```python
from build123d import *

# Parameters (mm, degrees)
BOSS_EXTRUDE3_DEPTH = 159.5
SHELL1_T            = -2.5
SKETCH1_W           = 154.5
SKETCH1_H           = 67.5
CUT_EXTRUDE2_DEPTH  = 4
CUT_EXTRUDE1_REACH  = 161.5
SKETCH2_W           = 4
SKETCH2_H           = 26
SKETCH8_W           = 179.5
SKETCH8_H           = 111.610999554
SKETCH8_W_2         = 159.5
SKETCH8_H_2         = 91.610999554
CUT_EXTRUDE3_DEPTH  = 56.944109771
SKETCH10_W          = 31.5
SKETCH10_H          = 55
CUT_EXTRUDE4_DEPTH  = 2.5
BOSS_EXTRUDE4_DEPTH = 13
CUT_EXTRUDE5_DEPTH  = 3.302
SKETCH13_R          = 2.6
CUT_EXTRUDE6_DEPTH  = 2.5
BOSS_EXTRUDE5_DEPTH = 1.6
SKETCH15_R          = 4
SKETCH15_R_2        = 1.4
BOSS_EXTRUDE6_DEPTH = 3
CUT_EXTRUDE7_REACH  = 6.236
SKETCH15_2_R        = 1.4


with BuildPart() as part:
    # Sketch3 → Boss-Extrude3 (new body)
    with BuildSketch(Plane.YZ.offset(-81.169946448)):
        Polygon((37, 0), (50.833221776, -14.444444444), (7.499888442, -55.944109771), (-40.777777778, -5.53328871), (-35, 0), align=None)
    extrude(amount=BOSS_EXTRUDE3_DEPTH)

    # Shell1
    shell1_openings = [part.faces().sort_by_distance(p)[0] for p in [
        (-1.419946448, 1, 0),
    ]]
    offset(amount=SHELL1_T, openings=shell1_openings, kind=Kind.INTERSECTION)

    # Sketch1 → Cut-Extrude2 (cut)
    with BuildSketch(Plane.XY):
        with Locations((-1.419946448, 0.902066229)):
            Rectangle(SKETCH1_W, SKETCH1_H)
    extrude(amount=-CUT_EXTRUDE2_DEPTH, mode=Mode.SUBTRACT)

    # Sketch2 → Cut-Extrude1 (cut, up to next)
    with BuildSketch(Plane.ZY.offset(81.169946448), mode=Mode.PRIVATE) as cut_extrude1_sk1:
        with Locations((-15.25, -1.097933771)):
            Rectangle(SKETCH2_W, SKETCH2_H)
    cut_extrude1_tool1 = extrude(cut_extrude1_sk1.sketch, amount=-CUT_EXTRUDE1_REACH, mode=Mode.PRIVATE) & part.part
    add(cut_extrude1_tool1.solids().sort_by_distance((-81.169946, -1.097934, -15.25))[0], mode=Mode.SUBTRACT)

    # Sweep1: sweep along a path in Sketch6
    with BuildLine(Plane.XY.offset(-1.8)) as sweep1_path:
        Line((-78.669946448, 34.652066229), (75.830053552, 34.652066229))
        Line((75.830053552, 34.652066229), (75.830053552, -32.847933771))
        Line((75.830053552, -32.847933771), (-78.669946448, -32.847933771))
        Line((-78.669946448, -32.847933771), (-78.669946448, 34.652066229))
    # Sketch7 → Sweep1 (sweep)
    with BuildSketch(Plane.ZY.offset(-75.830053552)):
        Polygon((-1.356838972, 35.114808383), (-2.636411987, 33.778697272), (-4.236411987, 33.778697272), (-4.236411987, 37.872531068), align=None)
    sweep(path=sweep1_path.line, transition=Transition.RIGHT)

    # Sketch8 → Cut-Extrude3 (cut, through all)
    with BuildSketch(Plane.XY):
        with Locations((-1.419946448, 5.027721999)):
            Rectangle(SKETCH8_W, SKETCH8_H)
        with Locations((-1.419946448, 5.027721999)):
            Rectangle(SKETCH8_W_2, SKETCH8_H_2, mode=Mode.SUBTRACT)
    extrude(amount=-CUT_EXTRUDE3_DEPTH, mode=Mode.SUBTRACT)

    # Sketch10 → Cut-Extrude4 (cut)
    with BuildSketch(Plane(origin=(0, 31.533839059, -32.927165761), x_dir=(-1, 0, 0), z_dir=(0, 0.691661089, -0.722222222))):
        with Locations((62.919946448, -3.277777778)):
            Rectangle(SKETCH10_W, SKETCH10_H)
    extrude(amount=-CUT_EXTRUDE4_DEPTH, mode=Mode.SUBTRACT)

    # Sketch10<3> → Boss-Extrude4 (add)
    with BuildSketch(Plane(origin=(0, 31.533839059, -32.927165761), x_dir=(-1, 0, 0), z_dir=(0, 0.691661089, -0.722222222))):
        Polygon((78.669946448, 24.222222222), (78.669946448, -30.777777778), (47.169946448, -30.777777778), (47.169946448, -33.277777778), (81.169946448, -33.277777778), (81.169946448, 26.722222222), (47.169946448, 26.722222222), (47.169946448, 24.222222222), align=None)
    extrude(amount=BOSS_EXTRUDE4_DEPTH)

    # Sketch12 → Cut-Extrude5 (cut)
    with BuildSketch(Plane(origin=(0, 31.533839059, -32.927165761), x_dir=(-1, 0, 0), z_dir=(0, 0.691661089, -0.722222222))):
        Polygon((47.169946448, -33.277777778), (-15.830053552, -33.277777778), (-15.830053552, -13.277777778), (24.169946448, 26.722222222), (47.169946448, 26.722222222), align=None)
    extrude(amount=-CUT_EXTRUDE5_DEPTH, mode=Mode.SUBTRACT)

    # Sketch13 → Cut-Extrude6 (cut)
    with BuildSketch(Plane(origin=(0, 31.533839059, -32.927165761), x_dir=(-1, 0, 0), z_dir=(0, 0.691661089, -0.722222222))):
        with Locations((-68.330053552, -23.277777778)):
            Circle(SKETCH13_R)
        with Locations((-33.330053552, -23.277777778)):
            Circle(SKETCH13_R)
        with Locations((-33.330053552, 16.722222222)):
            Circle(SKETCH13_R)
        with Locations((1.669946448, 16.722222222)):
            Circle(SKETCH13_R)
        with Locations((-68.330053552, 16.722222222)):
            Circle(SKETCH13_R)
    extrude(amount=-CUT_EXTRUDE6_DEPTH, mode=Mode.SUBTRACT)

    # Sketch14 → Boss-Extrude5 (add)
    with BuildSketch(Plane(origin=(0, 0, -4.236411987), x_dir=(-1, 0, 0), z_dir=(0, 0, -1))):
        with BuildLine():
            Line((77.796577491, -31.974564814), (67.796577491, -31.974564814))
            Line((67.796577491, -31.974564814), (67.796577491, -27.974564814))
            ThreePointArc((67.796577491, -27.974564814), (68.968150366, -25.14613769), (71.796577491, -23.974564814))
            Line((71.796577491, -23.974564814), (77.796577491, -23.974564814))
            Line((77.796577491, -23.974564814), (77.796577491, -31.974564814))
        make_face()
        with BuildLine():
            Line((-74.956684595, -31.974564814), (-64.956684595, -31.974564814))
            Line((-64.956684595, -31.974564814), (-64.956684595, -27.974564814))
            ThreePointArc((-64.956684595, -27.974564814), (-66.12825747, -25.14613769), (-68.956684595, -23.974564814))
            Line((-68.956684595, -23.974564814), (-74.956684595, -23.974564814))
            Line((-74.956684595, -23.974564814), (-74.956684595, -31.974564814))
        make_face()
    extrude(amount=-BOSS_EXTRUDE5_DEPTH)

    # Sketch15 → Boss-Extrude6 (add)
    with BuildSketch(Plane(origin=(0, 0, -4.236411987), x_dir=(-1, 0, 0), z_dir=(0, 0, -1))):
        with Locations((71.796577491, -27.974564814)):
            Circle(SKETCH15_R)
        with Locations((71.796577491, -27.974564814)):
            Circle(SKETCH15_R_2, mode=Mode.SUBTRACT)
        with Locations((-68.956684595, -27.974564814)):
            Circle(SKETCH15_R)
        with Locations((-68.956684595, -27.974564814)):
            Circle(SKETCH15_R_2, mode=Mode.SUBTRACT)
    extrude(amount=BOSS_EXTRUDE6_DEPTH)

    # Sketch15<2> → Cut-Extrude7 (cut, up to next)
    with BuildSketch(Plane(origin=(0, 0, -4.236411987), x_dir=(-1, 0, 0), z_dir=(0, 0, -1)), mode=Mode.PRIVATE) as cut_extrude7_sk1:
        with Locations((71.796577491, -27.974564814)):
            Circle(SKETCH15_2_R)
    cut_extrude7_tool1 = extrude(cut_extrude7_sk1.sketch, amount=-CUT_EXTRUDE7_REACH, mode=Mode.PRIVATE) & part.part
    add(cut_extrude7_tool1.solids().sort_by_distance((-71.796577, -27.974565, -4.236412))[0], mode=Mode.SUBTRACT)
    # Sketch15<2> → Cut-Extrude7 (cut, up to next)
    with BuildSketch(Plane(origin=(0, 0, -4.236411987), x_dir=(-1, 0, 0), z_dir=(0, 0, -1)), mode=Mode.PRIVATE) as cut_extrude7_sk2:
        with Locations((-68.956684595, -27.974564814)):
            Circle(SKETCH15_2_R)
    cut_extrude7_tool2 = extrude(cut_extrude7_sk2.sketch, amount=-CUT_EXTRUDE7_REACH, mode=Mode.PRIVATE) & part.part
    add(cut_extrude7_tool2.solids().sort_by_distance((68.956685, -27.974565, -4.236412))[0], mode=Mode.SUBTRACT)


solid = part.part
```
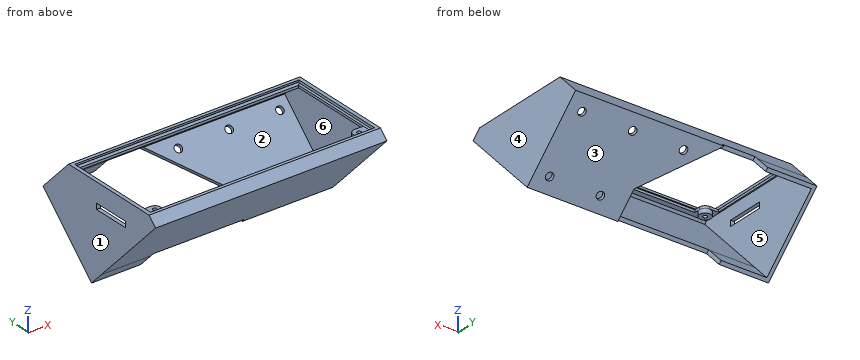
The listing builds one solid part. Answer for the finished solid, in the listing's coordinates (mm). Face numbers are marked on the shaded views. A direction names the side the tool comes from. Give positions to 0.01 mm unless a question says otherwise; leave off trailing zeros. Loops run counter-clockwise (first coordinate to the right, second up) from the corner with the lowest first, then second, coordinate; pieces in that order, holes last. Notation, with made-up numbers: (42, 32.25) - (73, 32.25) arc R14 cw to (73, 39.25) - close; hole circle Ø9 at (-14, 36). An arc over 180 degrees is marked (long way). Return JSON: item names as keys, results as strings. Group by question number.
1. Find section B-B (y = -1). Write down the section's boundary in (x, z), then the cut area to 3 significant figures.
2. Determine the mould class of the marked faces 3, 4, 5 and 6 for opening direction Z: pulls with the +Z half, pulls with the -Z half, needs draft (parallel to the pull), parting line crosses it, or undercut.
3. Which of the six approach directions +Z, -Z, +X, -X, +Y, -Y give full straight-line access (tool end or side, diameter ignored) to the marked faces 1 and 2?
4. Find section A-A (x = -34). Write down the section's boundary in (y, z), then the cut area to 3 significant figures.
5. Straight lines are drawn through the part: line 1 (X direction, y = 5, z = -7); line 2 (Y direction, x = 53.5, z = -16); line 3 (X direction, y = 15.5, z = -58.5). For each, find the intervals that lie inside material, in ascending order. Write a range as [from, to].
6. Given pin 1 Ø6 at (x, z) = (-29.5, -50.5) entering from +Y; pin 2 Ø1.5 at (x, y) = (1, 6.5) entering from -Z; pin 3 Ø2.5 at (x, y) = (-72, -29.5) entering from -Z, each flat-ended and moving along its own axis, determine where each tip first touches the part or whether it passes through.
7. Find section D-D (z = -36). Write down the section's boundary in (x, y).
8. Find section C-C (x = 55.5). Write down the section's boundary in (y, z).
Verdict:
{
 "1": {"outline": "(-81.17, -47.07) - (78.33, -47.07) - (78.33, 0) - (75.83, 0) - (75.83, -1.8) - (74.96, -2.64) - (74.96, -4.24) - (75.83, -4.24) - (75.83, -43.45) - (-78.67, -43.45) - (-78.67, -17.25) - (-81.17, -17.25) - close; (-81.17, -13.25) - (-78.67, -13.25) - (-78.67, -4.24) - (-77.8, -4.24) - (-77.8, -2.64) - (-78.67, -1.8) - (-78.67, 0) - (-81.17, 0) - close", "area": "787 mm^2"},
 "2": {"face 3": "pulls with the -Z half", "face 4": "needs draft", "face 5": "undercut", "face 6": "undercut"},
 "3": {"face 1": "+Z, -Z, -X, +Y, -Y", "face 2": "none"},
 "4": {"outline": "(-40.78, -5.53) - (5.22, -53.56) - (7.02, -51.83) - (-37.24, -5.61) - (-35.81, -4.24) - (-31.97, -4.24) - (-31.97, -2.64) - (-33.06, -1.6) - (-32.85, -1.4) - (-32.85, 0) - (-35, 0) - close; (33.78, -4.24) - (37.6, -4.24) - (46.74, -13.79) - (48.55, -12.06) - (37, 0) - (34.65, 0) - (34.65, -1.16) - (34.97, -1.5) - (33.78, -2.64) - close", "area": "238 mm^2"},
 "5": {"line 1": "x = [-81.17, -78.67], [75.83, 78.33]", "line 2": "y = [-30.75, -27.29], [45.59, 49.21]", "line 3": "x = [-81.17, -78.67]"},
 "6": {"pin 1": "stops at y = 7.02", "pin 2": "stops at z = -53.05", "pin 3": "stops at z = -18.61"},
 "7": {"outline": "(-81.17, -11.6) - (78.33, -11.6) - (78.33, 28.33) - (6.99, 28.33) - (9.61, 24.71) - (75.83, 24.71) - (75.83, -8.14) - (-78.67, -8.14) - (-78.67, 47.12) - (-81.17, 47.12) - close"},
 "8": {"outline": "(-40.78, -5.53) - (7.5, -55.94) - (50.83, -14.44) - (37, 0) - (34.65, 0) - (34.65, -1.16) - (34.97, -1.5) - (33.78, -2.64) - (33.78, -4.24) - (37.6, -4.24) - (47.3, -14.37) - (7.58, -52.41) - (-37.24, -5.61) - (-35.81, -4.24) - (-31.97, -4.24) - (-31.97, -2.64) - (-33.06, -1.6) - (-32.85, -1.4) - (-32.85, 0) - (-35, 0) - close"}
}
